from build123d import *

# Parameters (mm, degrees)
BOSS_EXTRUDE1_DEPTH = 500
CUT_EXTRUDE1_DEPTH  = 1000
CUT_EXTRUDE2_DEPTH  = 1000
SKETCH5_W           = 533.4
SKETCH5_H           = 228.6
SKETCH5_W_2         = 508
SKETCH5_H_2         = 203.2
BOSS_EXTRUDE2_DEPTH = 3.175
SKETCH6_W           = 152.4
SKETCH6_H           = 375
CUT_EXTRUDE4_DEPTH  = 381
BOSS_EXTRUDE4_DEPTH = 76.2


with BuildPart() as part:
    # Sketch2 → Boss-Extrude1 (new, symmetric)
    with BuildSketch(Plane(origin=(0, 0, 0), x_dir=(0, 0, -1), z_dir=(1, 0, 0))):
        Polygon((0, -750), (-500, -750), (-500, -288.675134595), (-118.676951522, -68.518169908), (0, -375), align=None)
    extrude(amount=BOSS_EXTRUDE1_DEPTH, both=True)

    # Sketch3 → Cut-Extrude1 (cut)
    with BuildSketch(Plane.XZ.offset(750)):
        with BuildLine():
            Line((-161.921680379, 500), (-500, 500))
            Line((-500, 500), (-500, 0))
            Line((-500, 0), (-375, 0))
            add(Edge.make_bspline(
                [(-375, 0), (-359.934223317, 289.431587022), (-161.921680379, 500)],
                knots=[0, 0, 0, 1, 1, 1], degree=2))
        make_face()
        with BuildLine():
            Line((500, 0), (500, 500))
            Line((500, 500), (161.921680379, 500))
            add(Edge.make_bspline(
                [(375, 0), (359.934223317, 289.431587022), (161.921680379, 500)],
                knots=[0, 0, 0, 1, 1, 1], degree=2))
            Line((375, 0), (500, 0))
        make_face()
    extrude(amount=-CUT_EXTRUDE1_DEPTH, mode=Mode.SUBTRACT)

    # Sketch4 → Cut-Extrude2 (cut)
    with BuildSketch(Plane(origin=(0, 0, 0), x_dir=(-1, 0, 0), z_dir=(0, 0, -1))):
        with BuildLine():
            Line((-375, -375), (-996.294304176, -375))
            Line((-996.294304176, -375), (-996.294304176, 371.909901341))
            Line((-996.294304176, 371.909901341), (846.489564783, 371.909901341))
            Line((846.489564783, 371.909901341), (846.489564783, -375))
            Line((846.489564783, -375), (375, -375))
            add(Edge.make_bspline(
                [(-375, -375), (0, 724.407090278), (375, -375)],
                knots=[0, 0, 0, 1, 1, 1], degree=2))
        make_face()
    extrude(amount=-CUT_EXTRUDE2_DEPTH, mode=Mode.SUBTRACT)

    # Sketch5 → Boss-Extrude2 (add)
    with BuildSketch(Plane(origin=(0, -48.896596526, 126.274884856), x_dir=(-1, 0, 0), z_dir=(0, 0.36109683475385423, -0.9325283244656689))):
        with Locations((0, -187.918797542)):
            Rectangle(SKETCH5_W, SKETCH5_H)
        with Locations((0, -187.918797542)):
            Rectangle(SKETCH5_W_2, SKETCH5_H_2, mode=Mode.SUBTRACT)
    extrude(amount=BOSS_EXTRUDE2_DEPTH)

    # Sketch6 → Cut-Extrude4 (cut)
    with BuildSketch(Plane(origin=(0, 0, 0), x_dir=(-1, 0, 0), z_dir=(0, 0, -1))):
        with Locations((-177.8, -562.5)):
            Rectangle(SKETCH6_W, SKETCH6_H)
        with Locations((177.8, -562.5)):
            Rectangle(SKETCH6_W, SKETCH6_H)
    extrude(amount=-CUT_EXTRUDE4_DEPTH, mode=Mode.SUBTRACT)

    # Sketch7 → Boss-Extrude4 (add, symmetric)
    with BuildSketch(Plane(origin=(0, 0, 0), x_dir=(0, 0, -1), z_dir=(1, 0, 0))):
        Polygon((0, -375), (152.4, -566.804213416), (152.4, -750), (0, -750), align=None)
    extrude(amount=BOSS_EXTRUDE4_DEPTH, both=True)


solid = part.part
Geometry: final body of the model. Coordinates: model frame, mm. A direction names the side the tool comes from. Give positions to 0.01 mm unless a question says otherwise; leave off trailing zeros. Write each loop counter-clockwise with the first axis right and the second up, starting at its lowest first coordinate (ties: lowest second). Pieces come first, ordered by that corner, then holes. Notation, with made-up numbers: M -21.5,32.5 L 8.5,32.5 A13 ccw 8.5,43.5 Z; hole C 8,65.5 d11. An arc over 180 degrees is marked long. Answer in a Markdown table with one row per item. Add a question column.
(1) Mould query, pull axis X, two halves, no side actions, for faces 4 (the flat face through (-266.7, -225, 56)), 5 (the flat face through (5, -750, 242)), 6 (the flat face through (-254, -225, 56)), 7 (the flat face through (254, -565, 188)). Classes: +X half, -X half, draft (parallel to the pull), parting line (faces both ways), or undercut.
(2) Section B-B on z = -93. Return loops of the section in (x, y), and give its area (3 significant figures).
(3) Ray query, line 1 (X direction, y = -583.5, z = 235); line 2 (X direction, y = -582, z = 196); line 3 (Z direction, x = -145, y = -599.5). Return the intervals inside material, ascending.
(4) Section C-C on x = -126. Return loops of the section in (y, z).
(5) Reachability of faces 1 (the flat face through (266.7, -225, 56)), 2 (the flat face through (179, -560, 381)), 3 (the flat face through (76.2, -602, -77)) from +Z, -Z, +X, -X, +Y, -Y: full face, straight path, thin tool, end or side. Return the list, or none.
(6) First-contact query: pin 1 (4 mm diameter, centred on y = -303.5, z = 158.5, fed in from -X); pin 2 (10 mm diameter, centred on x = 12, y = -183, fed in from +Z); pin 3 (5 mm diameter, centred on x = 177.5, z = 16.5, fed in from +Y); pin 4 (23 mm diameter, centred on y = -212, z = 45, fed in from -X). Flat tips, straight axial feed; report the tip coordinate or a pass-through.
(7) Section A-A on x = 35. Return loops of the section in (y, z), and give its area (3 significant figures).
Result set:
| question | item | result |
|---|---|---|
| 1 | face 4 | -X half |
| 1 | face 5 | draft |
| 1 | face 6 | undercut |
| 1 | face 7 | undercut |
| 2 | outline | M -76.2,-750 L 76.2,-750 L 76.2,-492.05 L -76.2,-492.05 Z |
| 2 | area | 39,300 mm^2 |
| 3 | line 1 | x = -327.97 to -254, -101.6 to 101.6, 254 to 327.97 |
| 3 | line 2 | x = -341.11 to -254, -101.6 to 101.6, 254 to 341.11 |
| 3 | line 3 | z = 381 to 500 |
| 4 | outline | M -750,381 L -375,381 L -375,0 L -330.72,17.14 L -329.58,14.18 L -317.73,18.77 L -318.88,21.73 L -129.39,95.11 L -128.24,92.14 L -116.4,96.73 L -117.55,99.69 L -68.52,118.68 L -288.68,500 L -750,500 Z |
| 5 | face 1 | -Z, +X, +Y |
| 5 | face 2 | -Z, -Y |
| 5 | face 3 | -Z, +X, +Y, -Y |
| 6 | pin 1 | stops at x = -350.49 |
| 6 | pin 2 | stops at z = 325.63 |
| 6 | pin 3 | stops at y = -317.73 |
| 6 | pin 4 | passes through |
| 7 | outline | M -750,-152.4 L -566.8,-152.4 L -375,0 L -330.72,17.14 L -329.58,14.18 L -317.73,18.77 L -318.88,21.73 L -129.39,95.11 L -128.24,92.14 L -116.4,96.73 L -117.55,99.69 L -68.52,118.68 L -288.68,500 L -750,500 Z |
| 7 | area | 323,000 mm^2 |
